Part model, mm, in its own coordinate system. Give positions to 0.01 mm unless a question says otherwise; leave off trailing zeros. Order: outer loops, then holes, each group sorted by start corner. A loop starts at its lowest first (then second) coordinate and runs counter-clockwise, first axis right, second up.
1. Slice it at B-B on y = -12.5. List the corners of the cut face in (x, z), and give its area (3 significant figures).
2. Slice it at A-A on x = -112.5. List the corners of the cut face in (y, z), and give its area (3 significant figures).
3. Slice it at C-C on z = 9.5. Give the number of separate pieces and of enclosed holes in the cut face, and give its area (3 significant figures).
4. Probe line 1 (Y direction, x = 60, z = 4.5); line 2 (Y direction, x = 138, z = 9); line 3 (X direction, y = 56, z = 11.5). List the from-to ranges inside material, lowest first.
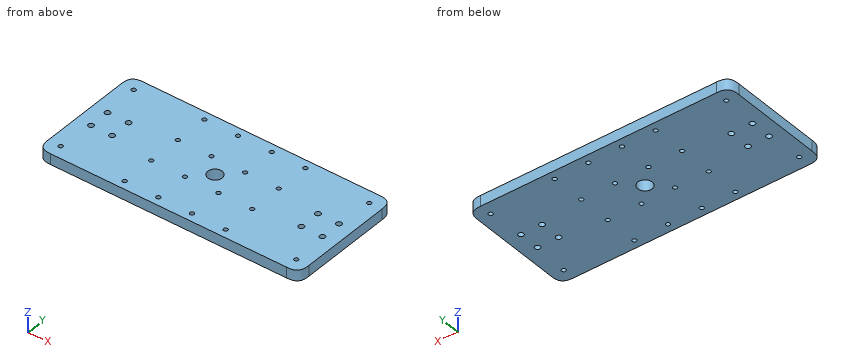
from build123d import *

# Parameters (mm, degrees)
SKETCH1_W                           = 310
SKETCH1_H                           = 140
BOSS_EXTRUDE1_DEPTH                 = 12.7
TAP_DRILL_FOR_M6X1_0_TAP1_D         = 5
LPATTERN1_COUNT                     = 4
LPATTERN1_PITCH                     = 40
LPATTERN1_COUNT_DIR2                = 4
LPATTERN1_PITCH_DIR2                = 40
FILLET1_SIZE                        = 15
M6_CLEARANCE_HOLE1_D                = 6.4
M16_CLEARANCE_HOLE1_D               = 17
TAP_START                           = -1
TAP_DRILL_FOR_M6X1_0_TAP2_OUTLINE_R = 2.5
TAP_DRILL_FOR_M6X1_0_TAP2_DEPTH     = 15


with BuildPart() as part:
    # Sketch1 → Boss-Extrude1 (new body)
    with BuildSketch(Plane.XY):
        Rectangle(SKETCH1_W, SKETCH1_H)
    extrude(amount=BOSS_EXTRUDE1_DEPTH)

    # Tap Drill for M6x1.0 Tap1 (through all)
    with Locations(Plane.XY.offset(12.7)):
        with Locations((-60, 60)):
            tap_drill_for_m6x1_0_tap1 = Hole(TAP_DRILL_FOR_M6X1_0_TAP1_D / 2)

    # LPattern1: Tap Drill for M6x1.0 Tap1 4 × 4
    with Locations(*[(i * LPATTERN1_PITCH, -j * LPATTERN1_PITCH_DIR2, 0) for i in range(LPATTERN1_COUNT) for j in range(LPATTERN1_COUNT_DIR2) if (i, j) != (0, 0)]):
        add(tap_drill_for_m6x1_0_tap1, mode=Mode.SUBTRACT)

    # Fillet1
    # a fillet whose section is not a circle: 15 mm, written as the material it takes off along each edge
    with BuildSketch(Plane(origin=(155, -70, -37.5), x_dir=(0, 1, 0), z_dir=(0, 0, 1)), Plane(origin=(155, 70, -37.5), x_dir=(-1, 0, 0), z_dir=(0, 0, 1))) as fillet1_piece_1:
        with BuildLine():
            add(Edge.make_bspline([(FILLET1_SIZE, 0), (FILLET1_SIZE * 0.831801948466, 0), (FILLET1_SIZE * 0.663603896932, 0), (FILLET1_SIZE * 0.292893218813, FILLET1_SIZE * 0.0716919198361), (FILLET1_SIZE * 0.0716919198361, FILLET1_SIZE * 0.292893218813), (0, FILLET1_SIZE * 0.663603896932), (0, FILLET1_SIZE * 0.831801948466), (0, FILLET1_SIZE)], knots=[0, 0, 0, 0, 0, 0, 0.5, 0.5, 1, 1, 1, 1, 1, 1], degree=5))
            Line((0, FILLET1_SIZE), (0, 0))
            Line((0, 0), (FILLET1_SIZE, 0))
        make_face()
    extrude(amount=87.7, mode=Mode.SUBTRACT)
    with BuildSketch(Plane(origin=(-155, 70, -37.5), x_dir=(1, 0, 0), z_dir=(0, 0, 1)), Plane(origin=(-155, -70, -37.5), x_dir=(0, 1, 0), z_dir=(0, 0, 1))) as fillet1_piece_2:
        with BuildLine():
            add(Edge.make_bspline([(FILLET1_SIZE, 0), (FILLET1_SIZE * 0.831801948466, 0), (FILLET1_SIZE * 0.663603896932, 0), (FILLET1_SIZE * 0.292893218813, -FILLET1_SIZE * 0.0716919198361), (FILLET1_SIZE * 0.0716919198361, -FILLET1_SIZE * 0.292893218813), (0, -FILLET1_SIZE * 0.663603896932), (0, -FILLET1_SIZE * 0.831801948466), (0, -FILLET1_SIZE)], knots=[0, 0, 0, 0, 0, 0, 0.5, 0.5, 1, 1, 1, 1, 1, 1], degree=5))
            Line((0, -FILLET1_SIZE), (0, 0))
            Line((0, 0), (FILLET1_SIZE, 0))
        make_face()
    extrude(amount=87.7, mode=Mode.SUBTRACT)

    # M6 Clearance Hole1 (through all)
    with Locations(Plane(origin=(0, 0, 0), x_dir=(-1, 0, 0), z_dir=(0, 0, -1))):
        with Locations((137.5, -12.5), (137.5, 12.5), (112.5, 12.5), (112.5, -12.5), (-112.5, -12.5), (-137.5, -12.5), (-112.5, 12.5), (-137.5, 12.5)):
            Hole(M6_CLEARANCE_HOLE1_D / 2)

    # M16 Clearance Hole1 (through all)
    with Locations(Plane.XY.offset(12.7)):
        with Locations((0, 0)):
            Hole(M16_CLEARANCE_HOLE1_D / 2)

    # Tap Drill for M6x1.0 Tap2: read off the stored shape, not the designer's step
    # Tap Drill for M6x1.0 Tap2 outline → Tap Drill for M6x1.0 Tap2 (cut)
    with BuildSketch(Plane.XY.offset(TAP_START)):
        with Locations((140, 55)):
            Circle(TAP_DRILL_FOR_M6X1_0_TAP2_OUTLINE_R)
        with Locations((-140, -55)):
            Circle(TAP_DRILL_FOR_M6X1_0_TAP2_OUTLINE_R)
        with Locations((140, -55)):
            Circle(TAP_DRILL_FOR_M6X1_0_TAP2_OUTLINE_R)
        with Locations((-140, 55)):
            Circle(TAP_DRILL_FOR_M6X1_0_TAP2_OUTLINE_R)
    extrude(amount=TAP_DRILL_FOR_M6X1_0_TAP2_DEPTH, mode=Mode.SUBTRACT)


solid = part.part
Data:
1. outline: (-155, 0) - (-140.7, 0) - (-140.7, 12.7) - (-155, 12.7) - close; (-134.3, 0) - (-115.7, 0) - (-115.7, 12.7) - (-134.3, 12.7) - close; (-109.3, 0) - (109.3, 0) - (109.3, 12.7) - (-109.3, 12.7) - close; (115.7, 0) - (134.3, 0) - (134.3, 12.7) - (115.7, 12.7) - close; (140.7, 0) - (155, 0) - (155, 12.7) - (140.7, 12.7) - close
1. area: 3,610 mm2
2. outline: (-70, 0) - (-15.7, 0) - (-15.7, 12.7) - (-70, 12.7) - close; (-9.3, 0) - (9.3, 0) - (9.3, 12.7) - (-9.3, 12.7) - close; (15.7, 0) - (70, 0) - (70, 12.7) - (15.7, 12.7) - close
2. area: 1,620 mm2
3. separate pieces: 1
3. enclosed holes: 29
3. area: 42,400 mm2
4. line 1: y = -70 to -62.5, -57.5 to -22.5, -17.5 to 17.5, 22.5 to 57.5, 62.5 to 70
4. line 2: y = -70 to -56.5, -53.5 to -15.66, -9.34 to 9.34, 15.66 to 53.5, 56.5 to 70
4. line 3: x = -155 to -142.29, -137.71 to 137.71, 142.29 to 155
